Geometry check sheet. Reference: the model listing, model coordinates, mm. Round coordinates to 2 decimals unless told otherwise and drop trailing zeros. Write each loop counter-clockwise with the first axis right and the second up, starting at its lowest first coordinate (ties: lowest second). Pieces come first, ordered by that corner, then holes.
Item 1: Cross-section at B-B (z = 14). Enter the section's corners in (x, y), then the cut area to 3 significant figures.
Item 2: Depth check by flat-ended pin: P1, Ø2, axis at y = 2, z = 15, coming from the +X side; P2, Ø0.7, axis at y = 0, z = 20.5, coming from the +X side; P3, Ø0.7, axis at y = 0.5, z = 20, coming from the -X side. Enter the tip coordinate at first touch or a pass-through.
Item 3: Cross-section at C-C (x = -3). Enter the section's corners in (y, z), then the cut area to 3 significant figures.
Item 4: Scan lines: probe 1 along Y at (x, z) = (0.5, 16); probe 2 along Z at (x, y) = (2, 2.5); probe 3 along Y at (x, z) = (-1.5, -8.5). Record each from-to range of solid material in increasing order.
Item 5: Cross-section at A-A (y = 0). Enter the section's corners in (x, z), then the cut area to 3 significant figures.
Item 6: Cross-section at D-D (y = -2.5). Enter the section's corners in (x, z).
from build123d import *

# Parameters (mm, degrees)
CUT_EXTRUDE1_DEPTH = 1.75


with BuildPart() as part:
    # Sketch2 → Revolve1 (revolve)
    with BuildSketch(Plane(origin=(0, 0, 0), x_dir=(0, 0, -1), z_dir=(1, 0, 0)), mode=Mode.PRIVATE) as revolve1_sk:
        with BuildLine():
            Line((-21.1, 0), (21.1, 0))
            Line((21.1, 0), (21.1, 1.44))
            Line((21.1, 1.44), (20.54, 2))
            Line((20.54, 2), (-18.9, 2))
            Line((-18.9, 2), (-18.9, 3.8))
            Line((-18.9, 3.8), (-19.23, 3.8))
            ThreePointArc((-19.23, 3.8), (-20.306499853, 3.047002626), (-21.1, 2))
            Line((-21.1, 2), (-21.1, 0))
        make_face()
    revolve(revolve1_sk.sketch.rotate(Axis((0, 0, 21.1), (0, 0, -1)), 180), axis=Axis((0, 0, 21.1), (0, 0, -1)))

    # Sketch3 → Cut-Extrude1 (cut)
    with BuildSketch(Plane.XY.offset(21.1)):
        Polygon((0, 1.443375673), (-1.25, 0.721687836), (-1.25, -0.721687836), (0, -1.443375673), (1.25, -0.721687836), (1.25, 0.721687836), align=None)
    extrude(amount=-CUT_EXTRUDE1_DEPTH, mode=Mode.SUBTRACT)

    # Cut-Extrude2 cone 1 section (through the dimple's axis) → Cut-Extrude2 (revolve, cut)
    with BuildSketch(Plane(origin=(0, 0, 21.1), x_dir=(0, -1, 0), z_dir=(1, 0, 0))):
        Polygon((0, 0), (1.443375673, 0), (0, 1.443375673), align=None)
    revolve(axis=Axis((0, 0, 21.1), (0, 0, -1)), mode=Mode.SUBTRACT)


solid = part.part
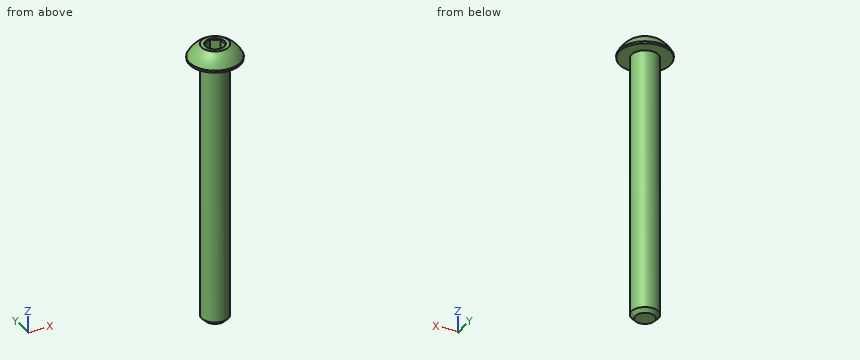
Resolved:
1. outline: circle Ø4 at (0, 0)
1. area: 12.6 mm2
2. P1: stops at x = 1.73
2. P2: stops at x = 3.19
2. P3: stops at x = -3.53
3. outline: (-2.33, 18.9) - (2.33, 18.9) - (2.33, 19.23) arc R2.98 ccw to (-2.33, 19.23) - close
3. area: 5.19 mm2
4. probe 1: y = -1.94 to 1.94
4. probe 2: z = 18.9 to 20.14
4. probe 3: y = -1.32 to 1.32
5. outline: (-3.8, 18.9) - (-2, 18.9) - (-2, -20.54) - (-1.44, -21.1) - (1.44, -21.1) - (2, -20.54) - (2, 18.9) - (3.8, 18.9) - (3.8, 19.23) arc R4.23 ccw to (2, 21.1) - (1.44, 21.1) - (1.25, 20.91) - (1.25, 19.35) - (-1.25, 19.35) - (-1.25, 20.91) - (-1.44, 21.1) - (-2, 21.1) arc R4.23 ccw to (-3.8, 19.23) - close
5. area: 169 mm2
6. outline: (-2.86, 18.9) - (2.86, 18.9) - (2.86, 19.23) arc R3.41 ccw to (-2.86, 19.23) - close
